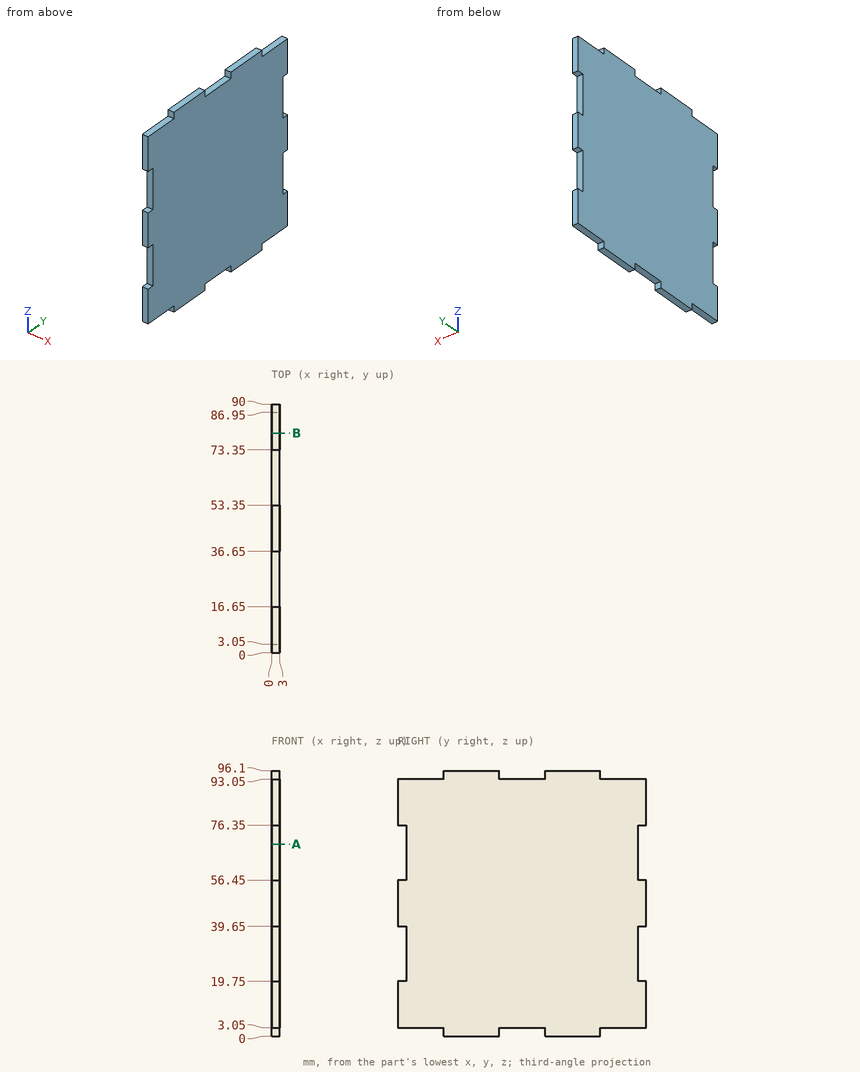
Here's the drawing with two shaded views (mm, measured from the low corner). I have some questions. Coordinates: 2 decimals unless noted, no trailing zeros. Write each loop counter-clockwise with the first axis right and the second up, starting at its lowest first coordinate (ties: lowest second). Pieces come first, ordered by that corner, then holes. Notation, with made-up numbers: (24, 22) - (34, 22) arc R21 ccw to (34, 61) - close; hole circle Ø6 at (-0.5, 39). An arc over 180 degrees is marked (long way). Return JSON: item names as keys, results as strings.
Q1. Please list where these lines run through material, in increasing order: L1, parallel to Y at x = 1.95, z = 22.5; L2, parallel to Z at x = 1.8, y = 48.5. Write a range as from..to.
Computed values:
{"L1": "y = 3.05..86.95", "L2": "z = 3.05..93.05"}
Q2. If we section it at A-A (z = 69.5): Please give me the cut outline in (x, y), then the cut area to 3 significant figures.
Computed values:
{"outline": "(0, 3.05) - (3, 3.05) - (3, 86.95) - (0, 86.95) - close", "area": "252 mm2"}
Q3. I'm going to push flat-ended pins straight in: pin 1 Ø1.5 at (x, z) = (1, 94.5) entering from +Y; pin 2 Ø0.9 at (x, z) = (1, 70) entering from -Y; pin 3 Ø0.9 at (x, y) = (2, 41) entering from -Z; pin 4 Ø1.5 at (x, z) = (1, 2.5) entering from -Y. Where does each tip first touch, or does it pass through?
Computed values:
{"pin 1": "stops at y = 73.35", "pin 2": "stops at y = 3.05", "pin 3": "stops at z = 3.05", "pin 4": "stops at y = 0"}
Q4. If we section it at B-B (y = 79.5): Please give me the cut outline in (x, z).
Computed values:
{"outline": "(0, 3.05) - (3, 3.05) - (3, 93.05) - (0, 93.05) - close"}
